Autodesk Fusion 360 part; units mm, degrees
sketch "Base" plane through (0, 0, 0) normal (0, 0, 1) x (1, 0, 0) in component "X Bearing Blocks"
  line L0 (12.8, 17.3) -> (-12.8, 17.3)
  line L1 (-12.8, 17.3) -> (-12.8, -17.3)
  line L2 (-12.8, -17.3) -> (12.8, -17.3)
  line L3 (12.8, -17.3) -> (12.8, 17.3)
  line L4 (12.8, 17.3) -> (-12.8, -17.3) construction
  line L5 (-12.8, 17.3) -> (12.8, -17.3) construction
  line L6 (-12.8, 0) -> (12.8, 0) construction
  line L7 (-12.8, 14.125) -> (12.8, 14.125)
  line L8 (-12.8, 9.875) -> (12.8, 9.875)
  line L9 (-12.8, 12) -> (12.8, 12) construction
  circle A0 centre (-8.5, 12) radius 2
  circle A1 centre (8.5, 12) radius 2
  line L10 (0, 17.3) -> (0, -17.3) construction
  line L11 (-12.8, -14.125) -> (12.8, -14.125)
  circle A2 centre (-8.5, -12) radius 2
  circle A3 centre (8.5, -12) radius 2
  line L12 (-12.8, -9.875) -> (12.8, -9.875)
  dimension "d484_1" = 25.6
  dimension "d485_1" = 34.6
  dimension "d489_1" = 4
  dimension "d490_1" = 4
  dimension "d491_1" = 12
  dimension "d492_1" = 17
  dimension "d493_1" = 8.5
  dimension "d495_1" = 2.125
  dimension "d496_1" = 2.125
extrude "Extrude1" add sketch "Base" along normal blind 21 contours L0 L1 L3 L7 | L1 L3 L7 L8 | L1 L3 L8 L12 | L1 L3 L11 L12 | L1 L2 L3 L11 | A0 | A1 | A2 | A3 in component "X Bearing Blocks"
sketch "Face" plane through (12.8, 0, 0) normal (1, 0, 0) x (0, 1, 0) in component "X Bearing Blocks"
  line L0 (-17.3, 0) -> (17.3, 0)
  line L1 (17.3, 0) -> (17.3, 21)
  line L2 (17.3, 21) -> (-17.3, 21)
  line L3 (-17.3, 21) -> (-17.3, 0)
  line L4 (0, 0) -> (0, 21) construction
  circle A0 centre (0, 11.5) radius 7.5
  circle A1 centre (0, 11.5) radius 4
  line L5 (-17.3, 0) -> (-17.3, 7.3)
  line L6 (-17.3, 7.3) -> (-16.2, 7.3)
  line L7 (-16.2, 7.3) -> (-16.2, 17.2)
  line L8 (-16.2, 17.2) -> (-11.55, 17.2)
  line L9 (17.3, 0) -> (17.3, 7.3)
  line L10 (17.3, 7.3) -> (16.2, 7.3)
  line L11 (16.2, 7.3) -> (16.2, 17.2)
  line L12 (16.2, 17.2) -> (11.55, 17.2)
  arc A2 (11.55, 17.2) -> (-11.55, 17.2) centre (0, 11.5) ccw
  dimension "d499_1" = 15
  dimension "d500_1" = 8
  dimension "d501_1" = 11.5
  dimension "d504_1" = 1.1
  dimension "d505_1" = 7.3
  dimension "d506_1" = 5.75
  dimension "d507_1" = 17.2
extrude "Extrude2" cut sketch "Face" against normal blind 25.6 contours L2 L3 L6 L7 L8 A2 | L1 L2 L10 L11 L12 A2 | A1 in component "X Bearing Blocks"
extrude "Extrude3" add sketch "Face" along normal mid plane 45 from surface at -12.8 contours A0 in component "X Bearing Blocks"
extrude "Extrude4" cut sketch "Base" along normal blind 4 contours A0 | A1 | A2 | A3 in component "X Bearing Blocks"
thread "Thread1" in component "X Bearing Blocks"
thread "Thread2" in component "X Bearing Blocks"
thread "Thread3" in component "X Bearing Blocks"
thread "Thread4" in component "X Bearing Blocks"
component "X Bearing Blocks" placed x (1, 0, 0) y (0, 1, 0) z (0, 0, 1) at (0, 0, 0)
equation "d197_1 = 4 mm"
equation "d198_1 = 6.00 mm"
equation "d199_1 = 6.00 mm"
equation "d200_1 = 4.00 mm"
equation "d201_1 = 12 mm"
equation "d202_1 = 90.0 deg"
equation "d203_1 = 12 mm"
equation "d204_1 = 90.0 deg"
equation "d205_1 = 12 mm"
equation "d206_1 = 90.0 deg"
equation "d207_1 = 51 mm"
equation "d209_1 = 51 mm"
equation "d210_1 = 12 mm"
equation "d211_1 = 90.0 deg"
equation "d212_1 = 30.0 mm"
equation "d213_1 = 30.00 mm"
equation "d214_1 = 12 mm"
equation "d215_1 = 90.0 deg"
equation "d216_1 = 12 mm"
equation "d217_1 = 90.0 deg"
equation "d218_1 = 2 mm"
equation "d225_1 = ( 3.6 / 2 ) * 1 mm"
equation "d227_1 = -1.5875 mm"
equation "d228_1 = 0.0 deg"
equation "d229_1 = 5.00 mm"
equation "d250_1 = 1.5875 mm"
equation "d251_1 = 0.0 deg"
equation "d253_1 = 21 mm + ( ( 39 / 2 ) * 1 mm )"
equation "d260_1 = 360.0 deg"
equation "d261_1 = -1.5875 mm"
equation "d262_1 = 0.0 deg"
equation "d284_1 = -1.588 mm"
equation "d285_1 = 0.0 deg"
equation "d286_1 = 0.00 mm"
equation "d287_1 = 1.588 mm"
equation "d288_1 = 0.0 deg"
equation "d301_1 = -1.588 mm"
equation "d302_1 = 0.0 deg"
equation "d342_1 = ( 17 / 2 ) * 1 mm"
equation "d343_1 = ( 17 / 2 ) * 1 mm"
equation "d386_1 = 0.00 mm"
equation "d387_1 = 19.7 mm"
equation "d388_1 = 0.0 deg"
equation "d389_1 = 0.00 mm"
equation "d390_1 = 6 mm"
equation "d391_1 = 0.0 deg"
equation "d400_1 = ( 92 / 2 ) * 1 mm"
equation "d407_1 = 0.00 mm"
equation "d408_1 = 9 mm"
equation "d409_1 = 0.0 deg"
equation "d410_1 = 1.588 mm"
equation "d411_1 = 0.0 deg"
equation "d433_1 = ( 92 / 2 ) * 1 mm"
equation "d448_1 = 0.00 mm"
equation "d449_1 = 0.00 mm"
equation "d450_1 = 0.00 mm"
equation "d451_1 = 0.0 deg"
equation "d452_1 = 0.00 mm"
equation "d453_1 = 0.00 mm"
equation "d454_1 = 0.00 mm"
equation "d455_1 = 0.0 deg"
equation "d456_1 = 90 deg"
equation "d457_1 = 0.00 mm"
equation "d458_1 = 0.00 mm"
equation "d459_1 = 0.00 mm"
equation "d460_1 = 0.00 mm"
equation "d461_1 = 0.00 mm"
equation "d462_1 = 0.00 mm"
equation "d463_1 = 0.0 deg"
equation "d464_1 = 0.00 mm"
equation "d465_1 = 0.00 mm"
equation "d466_1 = 0.00 mm"
equation "d467_1 = 0.0 deg"
equation "d468_1 = -90 deg"
equation "d469_1 = 0.00 mm"
equation "d470_1 = 0.00 mm"
equation "d471_1 = 0.00 mm"
equation "d491_1 = ( 24 / 2 ) * 1 mm"
equation "d493_1 = ( 17 / 2 ) * 1 mm"
equation "d495_1 = ( 4.25 / 2 ) * 1 mm"
equation "d496_1 = ( 4.25 / 2 ) * 1 mm"
equation "d497_1 = 21 mm"
equation "d498_1 = 0.0 deg"
equation "d501_1 = ( 15 / 2 ) * 1 mm + 4 mm"
equation "d508_1 = 0.0 deg"
equation "d509_1 = -25.60 mm"
equation "d510_1 = ( 45 / 2 ) * 1 mm"
equation "d511_1 = 0.0 deg"
equation "d512_1 = 0.00 mm"
equation "d513_1 = 4.00 mm"
equation "d514_1 = 0.0 deg"
equation "d515_1 = 0.00 mm"
equation "d516_1 = 0.00 mm"
equation "d517_1 = 0.00 mm"
equation "d518_1 = 0.0 deg"
equation "d519_1 = 0.00 mm"
equation "d520_1 = 0.00 mm"
equation "d521_1 = 0.00 mm"
equation "d522_1 = 0.0 deg"
equation "d523_1 = 90 deg"
equation "d524_1 = 0.00 mm"
equation "d525_1 = 0.00 mm"
equation "d526_1 = 0.00 mm"
equation "d527_1 = 0.00 mm"
equation "d528_1 = 0.00 mm"
equation "d529_1 = 0.00 mm"
equation "d530_1 = 0.0 deg"
equation "d531_1 = 0.00 mm"
equation "d532_1 = 0.00 mm"
equation "d533_1 = 0.00 mm"
equation "d534_1 = 0.0 deg"
equation "d535_1 = 90 deg"
equation "d536_1 = 0.00 mm"
equation "d537_1 = 0.00 mm"
equation "d538_1 = 0.00 mm"
equation "d539_1 = 0.00 mm"
equation "d540_1 = 0.00 mm"
equation "d541_1 = 0.00 mm"
equation "d542_1 = 0.0 deg"
equation "d543_1 = 0.00 mm"
equation "d544_1 = 0.00 mm"
equation "d545_1 = 0.00 mm"
equation "d546_1 = 0.0 deg"
equation "d547_1 = 0.0 deg"
equation "d548_1 = 0.00 mm"
equation "d549_1 = 0.00 mm"
equation "d550_1 = 0.00 mm"
equation "d587_1 = 0.00 mm"
equation "d588_1 = 0.00 mm"
equation "d589_1 = 0.00 mm"
equation "d590_1 = 0.0 deg"
equation "d491_1 = ( 24 / 2 ) * 1 mm"
equation "d493_1 = ( 17 / 2 ) * 1 mm"
equation "d495_1 = ( 4.25 / 2 ) * 1 mm"
equation "d496_1 = ( 4.25 / 2 ) * 1 mm"
equation "d501_1 = ( 15 / 2 ) * 1 mm + 4 mm"
equation "d510_1 = ( 45 / 2 ) * 1 mm"
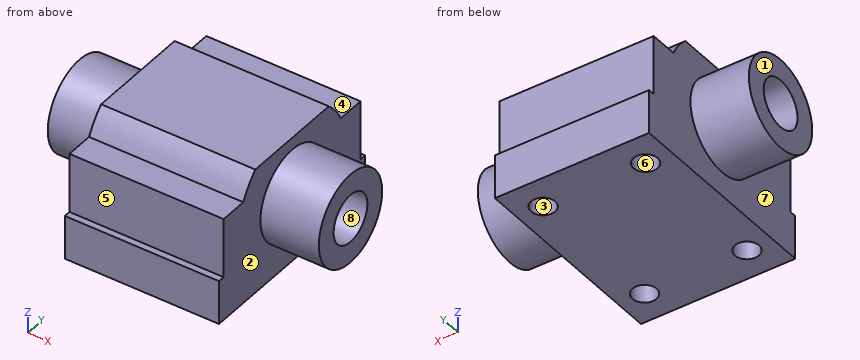
Check sheet for the modelled part. Datum: model origin and axes. Units: mm. Face numbers are marked on the shaded views. A direction names the side the tool comes from. Coordinates: 2 decimals unless noted, no trailing zeros. Order: outer loops, then holes, each group sorted by start corner. A loop starts at its lowest first (then second) coordinate and runs counter-clockwise, first axis right, second up. Notation, with made-up numbers: (-23, 47.5) -> (35, 47.5) arc R12 cw to (35, 60.5) -> close; hole circle Ø5 at (74.25, -12.75). An arc over 180 degrees is marked (long way). Write item = value, one per line. Start each with the question number.
1) Go/stop test with flat-tipped pins: P1, Ø3, axis at x = -8.5, y = 12, coming from the -Z side; P2, Ø5, axis at x = -1, y = 13, coming from the +Z side; P3, Ø2.5, axis at x = -0.5, y = -14, coming from the +Z side. Record where each tip stops, or that it passes through.
2) Material ranges on L1, parallel to Y at x = 8.5, z = 1.5; L2, parallel to X at y = 11, z = 2; L3, parallel to Z at x = 12, y = 0, recorded low to high.
3) Access from +Z, -Z, +X, -X, +Y, -Y to the whole of each face (thin tool, end or side, straight path). Record for the marked faces 1, 2, 3, 4 and 5.
4) Cross-section at D-D (x = -1.5). Enter the section's corners in (y, z).
5) Cross-section at B-B (x = -8.5). Enter the section's corners in (y, z).
6) Mould release check, pull along X, two halves, no side actions. Record for the marked faces 6, 7 and 8: +X half, -X half, draft (parallel to the pull), parting line (faces both ways), or undercut.
7) Cross-section at C-C (y = 11). Enter the section's corners in (x, z).
8) Cross-section at A-A (z = 11.5). Enter the section's corners in (x, y).
Ans:
q1.P1 = 4
q1.P2 = 18.96
q1.P3 = 17.2
q2.L1 = -17.3 to -14, -10 to 10, 14 to 17.3
q2.L2 = -12.8 to -10.23, -6.77 to 6.77, 10.23 to 12.8
q2.L3 = 0 to 7.5, 15.5 to 21
q3.face_1 = +Z, -Z, -X, +Y, -Y
q3.face_2 = +X
q3.face_3 = -Z
q3.face_4 = +Z, +X, -X, +Y
q3.face_5 = +Z, +X, -X, -Y
q4.outline = (-17.3, 0) -> (17.3, 0) -> (17.3, 7.3) -> (16.2, 7.3) -> (16.2, 17.2) -> (11.55, 17.2) arc R12.88 ccw to (8.7, 21) -> (-8.7, 21) arc R12.88 ccw to (-11.55, 17.2) -> (-16.2, 17.2) -> (-16.2, 7.3) -> (-17.3, 7.3) -> close; hole circle Ø8 at (0, 11.5)
q5.outline = (-17.3, 0) -> (-14, 0) -> (-14, 4) -> (-10, 4) -> (-10, 0) -> (10, 0) -> (10, 4) -> (14, 4) -> (14, 0) -> (17.3, 0) -> (17.3, 7.3) -> (16.2, 7.3) -> (16.2, 17.2) -> (11.55, 17.2) arc R12.88 ccw to (8.7, 21) -> (-8.7, 21) arc R12.88 ccw to (-11.55, 17.2) -> (-16.2, 17.2) -> (-16.2, 7.3) -> (-17.3, 7.3) -> close; hole circle Ø8 at (0, 11.5)
q6.face_6 = undercut
q6.face_7 = -X half
q6.face_8 = draft
q7.outline = (-12.8, 0) -> (-10.23, 0) -> (-10.23, 4) -> (-6.77, 4) -> (-6.77, 0) -> (6.77, 0) -> (6.77, 4) -> (10.23, 4) -> (10.23, 0) -> (12.8, 0) -> (12.8, 18.2) -> (-12.8, 18.2) -> close
q8.outline = (-22.5, -7.5) -> (-12.8, -7.5) -> (-12.8, -16.2) -> (12.8, -16.2) -> (12.8, -7.5) -> (22.5, -7.5) -> (22.5, -4) -> (-22.5, -4) -> close; (-22.5, 4) -> (22.5, 4) -> (22.5, 7.5) -> (12.8, 7.5) -> (12.8, 16.2) -> (-12.8, 16.2) -> (-12.8, 7.5) -> (-22.5, 7.5) -> close
